from build123d import *

# Parameters (mm, degrees)
SKETCH1_W           = 20.5
SKETCH1_H           = 15.5
BOSS_EXTRUDE1_DEPTH = 2
SKETCH3_W           = 10
SKETCH3_H           = 16
BOSS_EXTRUDE3_DEPTH = 11.5
SKETCH4_R           = 1.43812907
BOSS_EXTRUDE5_DEPTH = 1.5
CHAMFER1_SIZE       = 5


with BuildPart() as part:
    # Sketch1 → Boss-Extrude1 (new body)
    with BuildSketch(Plane(origin=(0, 0, 0), x_dir=(1, 0, 0), z_dir=(0, 1, 0))):
        Rectangle(SKETCH1_W, SKETCH1_H)
    extrude(amount=BOSS_EXTRUDE1_DEPTH)

    # Sketch3 → Boss-Extrude3 (add)
    with BuildSketch(Plane(origin=(0, 2, 0), x_dir=(1, 0, 0), z_dir=(0, 1, 0))):
        with Locations((0, 4.25)):
            Rectangle(SKETCH3_W, SKETCH3_H)
    extrude(amount=BOSS_EXTRUDE3_DEPTH)

    # Sketch4 → Boss-Extrude5 (add)
    with BuildSketch(Plane(origin=(0, 2, 0), x_dir=(1, 0, 0), z_dir=(0, 1, 0))):
        with Locations(Location((-8.644410723, 4.981189745, 0), (0, 0, 90))):
            Circle(SKETCH4_R)
    extrude(amount=BOSS_EXTRUDE5_DEPTH)

    # Chamfer1
    chamfer1_edges = [part.edges().sort_by_distance(p)[0] for p in [
        (0, 13.5, 3.75),
        (0, 13.5, -12.25),
    ]]
    chamfer(chamfer1_edges, length=CHAMFER1_SIZE)


solid = part.part
Read the model definition and answer for the solid it produces. Units are mm, in the model's axes. A direction names the side the tool comes from. Round coordinates to 2 decimals unless told otherwise and drop trailing zeros. Write each loop counter-clockwise with the first axis right and the second up, starting at its lowest first coordinate (ties: lowest second). Pieces come first, ordered by that corner, then holes.
1. Determine the mould class of faces 6 (the face through (10.25, 1, 0)), 7 (the face through (0, 5, -12.25)), 8 (the face through (-7.369, 2.74, -5.645)) for opening direction X: pulls with the +X half, pulls with the -X half, needs draft (parallel to the pull), parting line crosses it, or undercut.
2. Straight lines are drawn through the part: L1, parallel to Z at x = 0.75, y = 3.75; L2, parallel to Z at x = -4.25, y = 1; L3, parallel to Y at x = -8, z = -5.5. For each, find the intervals that lie inside material, in ascending order.
3. The part is cut by section C-C, the plane y = 10.5. Determine the outline of the cut face in (x, z).
4. The part is cut by section B-B, the plane x = -1.75. Determine the outline of the cut face in (y, z), then the cut area to 3 significant figures.
5. The part is cut by section A-A, the plane z = 0. Determine the outline of the cut face in (x, y).
6. Which of the six approach directions +Z, -Z, +X, -X, +Y, -Y give full straight-line access (tool end or side, diameter ignored) to faces 1 (the face through (-9, 3.5, -5)), 2 (the face through (0, 5, 3.75)), 3 (the face through (0, 0, 0)), 4 (the face through (5, 8, -4)), 5 (the face through (0, 1, -7.75))?
7. Given pin 1 Ø3 at (x, y) = (1, 6) entering from +Z; pin 2 Ø6 at (y, z) = (8.5, -7.5) entering from -X; pin 3 Ø5 at (y, z) = (8, 1) entering from +X, each flat-ended and moving along its own axis, determine where each tip first touches the part or whether it passes through.
8. The part is cut by section D-D, the plane z = -3.25. Determine the outline of the cut face in (x, y).
Values:
1. face 6: pulls with the +X half
1. face 7: needs draft
1. face 8: undercut
2. L1: z = -12.25 to 3.75
2. L2: z = -7.75 to 7.75
2. L3: y = 0 to 3.5
3. outline: (-5, -10.25) - (5, -10.25) - (5, 1.75) - (-5, 1.75) - close
4. outline: (0, -7.75) - (2, -7.75) - (2, -12.25) - (8.5, -12.25) - (13.5, -7.25) - (13.5, -1.25) - (8.5, 3.75) - (2, 3.75) - (2, 7.75) - (0, 7.75) - close
4. area: 190 mm2
5. outline: (-10.25, 0) - (10.25, 0) - (10.25, 2) - (5, 2) - (5, 12.25) - (-5, 12.25) - (-5, 2) - (-10.25, 2) - close
6. face 1: +Z, -Z, -X, +Y
6. face 2: +Z, +X, -X, +Y
6. face 3: +Z, -Z, +X, -X, -Y
6. face 4: +Z, -Z, +X, +Y
6. face 5: -Z, +X, -X, -Y
7. pin 1: stops at z = 3.75
7. pin 2: stops at x = -5
7. pin 3: stops at x = 5
8. outline: (-10.25, 0) - (10.25, 0) - (10.25, 2) - (5, 2) - (5, 13.5) - (-5, 13.5) - (-5, 2) - (-10.25, 2) - close
